Verification items for the finished model (mm, model axes). A direction names the side the tool comes from. Round coordinates to 2 decimals unless told otherwise and drop trailing zeros. Write each loop counter-clockwise with the first axis right and the second up, starting at its lowest first coordinate (ties: lowest second). Pieces come first, ordered by that corner, then holes. Notation, with made-up numbers: M 15,9 L 54,9 A22 ccw 54,31 Z; hole C -20.75,84.5 d1. An arc over 180 degrees is marked long. One line per question, with ' | ' between items.
from build123d import *

# Parameters (mm, degrees)
ENL_V_START                  = -8
ESQUISSE2_R                  = 3.1
ENL_V_MAT_EXTRU_1_DEPTH      = 30
R_P_TITION_CIRCULAIRE1_COUNT = 3
CONG_1_R                     = 15


with BuildPart() as part:
    # Esquisse1 → Révolution1 (revolve)
    with BuildSketch(Plane.XY, mode=Mode.PRIVATE) as r_volution1_sk:
        Polygon((7.5, 20), (0, 32.990381057), (0, 35.990381057), (17.5, 35.990381057), (17.5, 0), (7.5, 0), align=None)
    revolve(r_volution1_sk.sketch.rotate(Axis((0, 0, 0), (0, 1, 0)), 90), axis=Axis((0, 0, 0), (0, 1, 0)))

    # Esquisse2 → Enlèv. mat.-Extru.1 (cut)
    with BuildSketch(Plane.XY.offset(ENL_V_START)):
        with Locations((0, 5)):
            Circle(ESQUISSE2_R)
    enl_v_mat_extru_1 = extrude(amount=-ENL_V_MAT_EXTRU_1_DEPTH, mode=Mode.SUBTRACT)

    # Répétition circulaire1: Enlèv. mat.-Extru.1 ×3 about axis
    r_p_tition_circulaire1_axis = Axis((0, 0, 0), (0, 1, 0))
    for i in range(1, R_P_TITION_CIRCULAIRE1_COUNT):
        add(enl_v_mat_extru_1.rotate(r_p_tition_circulaire1_axis, i * 360 / R_P_TITION_CIRCULAIRE1_COUNT), mode=Mode.SUBTRACT)

    # Congé1
    cong_1_edges = [part.edges().sort_by_distance(p)[0] for p in [
        (0, 35.990381057, 17.5),
    ]]
    fillet(cong_1_edges, radius=CONG_1_R)


solid = part.part
1. Section check B-B, the plane y = 5. Record the cut outline in (x, z), then the cut area to 3 significant figures.
Results:
outline: M -16.47,5.93 A17.5 ccw -3.1,-17.22 L -3.1,-8 L 3.1,-8 L 3.1,-17.22 A17.5 ccw 16.47,5.93 L 8.48,1.32 L 5.38,6.68 L 13.37,11.3 A17.5 ccw -13.37,11.3 L -5.38,6.68 L -8.48,1.32 Z; hole C 0,0 d15 | area: 610 mm2
2. Mould release check, pull along Y, two halves, no side actions. Record for faces 1 (the face through (-0.86, 28.03, -2.73)), 2 (the face through (6.95, 5.04, 3.96)), 3 (the face through (-6.324, 10.14, -4.032)): pulls with the +Y half, pulls with the -Y half, needs draft (parallel to the pull), parting line crosses it, or undercut.
Results:
face 1: pulls with the -Y half | face 2: undercut | face 3: needs draft
3. Section check A-A, the plane y = 18. Record the cut outline in (x, z), then the cut area to 3 significant figures.
Results:
outline: C 0,0 d35; hole C 0,0 d15 | area: 785 mm2
4. Go/stop test with flat-tipped pins: P1, Ø2, axis at x = 0.5, z = -5, coming from the -Y side; P2, Ø2, axis at x = 7.5, y = 18.5, coming from the +Z side; P3, Ø1, axis at y = 9, z = 10.5, coming from the +X side. Record where each tip stops, or that it passes through.
Results:
P1: stops at y = 22.55 | P2: stops at z = 16.25 | P3: stops at x = 14.36
5. Tool access check on faces 4 (the face through (-6.907, 5.043, 4.038)), 5 (the face through (0, 5, -8)), 6 (the face through (17.084, 10.348, 3.794)). Record the directions out of +Z, -Z, +X, -X, +Y, -Y that give a thin tool (end or side, any length) a straight path to the whole face; none if there is none.
Results:
face 4: none | face 5: -Z | face 6: +Y, -Y
6. Thickness scan on line 1 (X direction, y = 15.75, z = 0); line 2 (Z direction, x = -6, y = 9.5); line 3 (Z direction, x = -11, y = 5). Record the ranges inside material, lowest first.
Results:
line 1: x = -17.5 to -7.5, 7.5 to 17.5 | line 2: z = -16.44 to -4.5, 4.5 to 16.44 | line 3: z = -13.61 to 2.77, 9.93 to 13.61
